Autodesk Fusion 360 part; units mm, degrees
sketch "Sketch1" plane through (0, 0, 0) normal (0, 0, 1) x (1, 0, 0)
  line L0 (36, 27) -> (-36, 27)
  line L1 (-36, 27) -> (-36, -27)
  line L2 (-36, -27) -> (36, -27)
  line L3 (36, -27) -> (36, 27)
  line L4 (36, 30.6) -> (-36, 30.6)
  line L5 (-36, 35.6) -> (-36, -30.6)
  line L6 (-36, -30.6) -> (36, -30.6)
  line L7 (36, -30.6) -> (36, 30.6)
  line L8 (33, 35.6) -> (-36, 35.6)
  line L9 (41, -27.6) -> (41, 27.6)
  line L10 (33, -35.6) -> (-36, -35.6)
  line L11 (-36, -35.6) -> (-36, 30.6)
  arc A0 (41, 27.6) -> (33, 35.6) centre (33, 27.6) ccw
  arc A1 (33, -35.6) -> (41, -27.6) centre (33, -27.6) ccw
  circle A2 centre (-31, 0) radius 1.75
  line L12 (-31, 11) -> (-10, 11)
  arc A3 (-10, 11) -> (-10, 19) centre (-10, 15) ccw
  line L13 (-10, 19) -> (-31, 19)
  arc A4 (-31, 19) -> (-31, 11) centre (-31, 15) ccw
  line L14 (-31, 15) -> (-10, 15) construction
  line L15 (1.75, 0) -> (22.5, 0)
  line L16 (-31, -11) -> (-10, -11)
  line L17 (-10, -19) -> (-31, -19)
  arc A5 (-10, -19) -> (-10, -11) centre (-10, -15) ccw
  arc A6 (-31, -11) -> (-31, -19) centre (-31, -15) ccw
  circle A7 centre (-10, 0) radius 1.75
  dimension "d1" = 72
  dimension "d2" = 54
  dimension "d3" = 61.2
  dimension "d6" = 8
  dimension "d32" = 3.5
  dimension "d34" = 8
  dimension "d40" = 3.5
extrude "Extrude1" add sketch "Sketch1" along normal blind 6.3 contours L3 L4 L5 L6 L7 L8 L9 L10 L11 A0 A1 | L0 L4 L5 L7 L11 | L2 L5 L6 L7 L11
extrude "Extrude2" add sketch "Sketch1" along normal blind 24 contours L3 L4 L5 L6 L7 L8 L9 L10 L11 A0 A1
extrude "Extrude3" add sketch "Sketch1" along normal blind 27 and the other way blind -24
sketch "Sketch2" plane through (0, -35.6, 0) normal (0, -1, 0) x (1, 0, 0)
  line L0 (-36, 0) -> (33, 0)
  line L1 (33, 0) -> (33, 27)
  line L2 (-36, 27) -> (-36, 0)
  line L3 (-36, 0) -> (-49.5029, 27)
  line L4 (-36, 0) -> (-6, 0) construction
  line L5 (-36, 27) -> (-49.5029, 27)
  line L6 (33, 27) -> (-36, 27)
  line L7 (-36, 27) -> (-36, 24)
  line L8 (-36, 24) -> (-36.4845, 24)
  line L9 (-36.4845, 24) -> (-48.0026, 24)
  line L10 (-36, 0) -> (-36, 6.4)
  line L11 (-36, 6.4) -> (-36, 6)
  line L12 (-36, 6.4) -> (-39.2007, 6.4)
  line L13 (-36, 0) -> (-32.4, 0)
  line L14 (-49.5029, 27) -> (-47.5029, 27)
  line L15 (-36, 6.4) -> (-32.4, 6.4)
  line L16 (-32.4, 6.4) -> (-32.4, 0)
  dimension "d11" = 116.57
  dimension "d25" = 6.4
  dimension "d36" = 3.6
  dimension "d37" = 2
extrude "Extrude4" add sketch "Sketch2" against normal blind 5 contours L2 L3 L10 L11 L12 | L2 L3 L8 L9 L12
extrude "Extrude5" add sketch "Sketch2" along normal blind -71.2 and the other way blind 66.2 contours L2 L3 L10 L11 L12 | L2 L3 L8 L9 L12
extrude "Extrude6" add sketch "Sketch2" against normal blind 71.2 contours L2 L3 L5 L7 L8 L9 L14
extrude "Extrude7" cut sketch "Sketch2" along normal blind -8.6 and the other way blind 5 contours L0 L2 L10 L11 L13 L15 L16
extrude "Extrude8" cut sketch "Sketch2" along normal blind -66.2 and the other way blind 62.6 contours L0 L2 L10 L11 L13 L15 L16
chamfer "Chamfer2" distance 1 angle 45 2 edges at (-32.6316, 0.6328, 24) (-11.6316, 0.6328, 24)
sketch "Sketch3" plane through (0, 0, 27) normal (0, 0, 1) x (-1, 0, 0)
  arc A0 (10, 19) -> (10, 11) centre (10, 15) ccw
  line L0 (10, 19) -> (31, 19)
  arc A1 (31, 11) -> (31, 19) centre (31, 15) ccw
  line L1 (31, 11) -> (10, 11)
  circle A2 centre (31, 0) radius 1.75
  circle A3 centre (10, 0) radius 1.75
  arc A4 (31, -19) -> (31, -11) centre (31, -15) ccw
  line L2 (31, -19) -> (10, -19)
  arc A5 (10, -11) -> (10, -19) centre (10, -15) ccw
  line L3 (10, -11) -> (31, -11)
  line L4 (49.5029, 35.6) -> (-33, 35.6)
  arc A6 (-33, 35.6) -> (-41, 27.6) centre (-33, 27.6) ccw
  line L5 (-41, 27.6) -> (-41, -27.6)
  arc A7 (-41, -27.6) -> (-33, -35.6) centre (-33, -27.6) ccw
  line L6 (-33, -35.6) -> (49.5029, -35.6)
  line L7 (49.5029, -35.6) -> (49.5029, 35.6)
  line L8 (2.0837, -40) -> (-45, -40)
  line L9 (-45, -40) -> (-45, 40)
  line L10 (-45, 40) -> (2.0837, 40)
  line L11 (2.0837, 40) -> (2.0837, -40)
extrude "Extrude9" cut sketch "Sketch3" against normal blind 55 contours L4 A6 L5 A7 L6 L11 | L4 A6 L5 A7 L6 L8 L9 L10 L11
chamfer "Chamfer3" distance 1 angle 45 2 edges at (-32.4, -28.8, 6.3) (-32.4, 28.8, 6.3)
Input: part model. Units: mm. Frame: model coordinates. A direction names the side the tool comes from. Coordinates: 2 decimals unless noted, no trailing zeros. Loops run counter-clockwise (first coordinate to the right, second up) from the corner with the lowest first, then second, coordinate; pieces in that order, holes last. Notation, with made-up numbers: (2, -38.75) -> (52, -38.75) arc R24 cw to (52, -4.75) -> close; hole circle Ø4 at (57, 32). An arc over 180 degrees is marked (long way). Use a Markdown table: item, result.
1) Cut plane A-A (x = -14). Return the cut outline in (y, z).
Results found:
| item | result |
|---|---|
| outline | (-35.6, 0) -> (-27, 0) -> (-27, 6.3) -> (-30.6, 6.3) -> (-30.6, 24) -> (-19, 24) -> (-19, 27) -> (-35.6, 27) -> close; (-11, 24) -> (11, 24) -> (11, 27) -> (-11, 27) -> close; (19, 24) -> (30.6, 24) -> (30.6, 6.3) -> (27, 6.3) -> (27, 0) -> (35.6, 0) -> (35.6, 27) -> (19, 27) -> close |
2) Pull-direction query (Y, two-part tool) for faces 5 (the flat face through (-20, -19, 25)), 6 (the flat face through (-19, 31, 0)), 7 (the flat face through (-21, 35.6, 14)); classes: released by +Y, released by -Y, zero draft, split by the parting line, or undercut.
Results found:
| item | result |
|---|---|
| face 5 | undercut |
| face 6 | zero draft |
| face 7 | released by +Y |
3) Access query for faces 1 (the flat face through (-17, 27, 3)), 2 (the flat face through (-17, 29, 6.3)), 3 (the flat face through (-32.4, -29, 3)), 4 (the flat face through (-21, 11, 25)). Directions: +Z, -Z, +X, -X, +Y, -Y. A direction counts if a zero-diameter tool reaches every point of the face in a straight line with its end or side. Return the directions, or none.
Results found:
| item | result |
|---|---|
| face 1 | -Z, +X, -X |
| face 2 | +X, -X |
| face 3 | -Z, -X |
| face 4 | +Z, -Z |
4) Contact query for flat-ended pins moving along their axis: pin 1 (1.8 mm diameter, centred on y = 28, z = 4, fed in from -X); pin 2 (4 mm diameter, centred on x = -19, y = -7, fed in from -Z). Output: stop coordinate, or through.
Results found:
| item | result |
|---|---|
| pin 1 | stops at x = -32.4 |
| pin 2 | stops at z = 24 |
5) Cut plane B-B (y = -13). Return the cut outline in (x, z), then the cut area to 3 significant figures.
Results found:
| item | result |
|---|---|
| outline | (-49.5, 27) -> (-48, 24) -> (-34.46, 24) -> (-34.46, 27) -> close; (-6.54, 24) -> (-2.08, 24) -> (-2.08, 27) -> (-6.54, 27) -> close |
| area | 56.2 mm2 |
6) Material intervals for line 1 along Y through (x, z) = (-31, 25.65); line 2 along Y through (x, z) = (-35.5, 3.25); line 3 along Y through (x, z) = (-14.5, 2.5), sorted ascending. Write a range as from..to.
Results found:
| item | result |
|---|---|
| line 1 | y = -35.6..-19, -11..-1.75, 1.75..11, 19..35.6 |
| line 2 | y = -35.6..-30.6, 30.6..35.6 |
| line 3 | y = -35.6..-27, 27..35.6 |
7) Cut plane C-C (z = 15.5). Return the cut outline in (x, y).
Results found:
| item | result |
|---|---|
| outline | (-43.75, -35.6) -> (-2.08, -35.6) -> (-2.08, -30.6) -> (-43.75, -30.6) -> close; (-43.75, 30.6) -> (-2.08, 30.6) -> (-2.08, 35.6) -> (-43.75, 35.6) -> close |
